```python
from build123d import *

# Parameters (mm, degrees)
CUT_EXTRUDE_1_DEPTH    = 6.35
CUT_EXTRUDE_START      = -12.7
CUT_EXTRUDE_2_DEPTH    = 12.7
HOLE_WIZARD_M2_1_D     = 2.3876
HOLE_WIZARD_M2_1_DEPTH = 4.7752
CHAMFER_1_SIZE         = 0.7874


with BuildPart() as part:
    # 스케치1 → 회전1 (revolve)
    with BuildSketch(Plane.XY, mode=Mode.PRIVATE) as revolve_1_sk:
        with BuildLine():
            Line((6.35, 38.1), (0, 38.1))
            Line((0, 38.1), (0, 0))
            Line((0, 0), (9.525, 0))
            Line((9.525, 0), (9.525, 13.263233373))
            ThreePointArc((9.525, 13.263233373), (9.110100453, 15.210106507), (7.9375, 16.818666364))
            ThreePointArc((7.9375, 16.818666364), (6.764899547, 18.42722622), (6.35, 20.374099354))
            Line((6.35, 20.374099354), (6.35, 38.1))
        make_face()
    revolve(revolve_1_sk.sketch.rotate(Axis((0, 38.1, 0), (0, -1, 0)), 270), axis=Axis((0, 38.1, 0), (0, -1, 0)))

    # 스케치2 → 컷-돌출1 (cut)
    with BuildSketch(Plane(origin=(0, 38.1, 0), x_dir=(-1, 0, 0), z_dir=(0, 1, 0))):
        with BuildLine():
            Line((-4.7498, -4.214486915), (-4.7498, 4.214486915))
            ThreePointArc((-4.7498, 4.214486915), (-6.35, 0), (-4.7498, -4.214486915))
        make_face()
    extrude(amount=-CUT_EXTRUDE_1_DEPTH, mode=Mode.SUBTRACT)

    # 스케치3 → 컷-돌출2 (cut)
    with BuildSketch(Plane.XZ.offset(CUT_EXTRUDE_START)):
        with BuildLine():
            Line((4.7498, -4.214486915), (4.7498, 4.214486915))
            ThreePointArc((4.7498, 4.214486915), (-6.35, 0), (4.7498, -4.214486915))
        make_face()
    extrude(amount=CUT_EXTRUDE_2_DEPTH, mode=Mode.SUBTRACT)

    # M2 여유 구멍1
    with Locations(Plane.ZY.offset(-4.7498)):
        with Locations((0, 6.35)):
            Hole(HOLE_WIZARD_M2_1_D / 2, depth=HOLE_WIZARD_M2_1_DEPTH)

    # 모따기1
    chamfer_1_edges = [part.edges().sort_by_distance(p)[0] for p in [
        (-5.791566796, 38.1, 2.603892095),
    ]]
    chamfer(chamfer_1_edges, length=CHAMFER_1_SIZE)


solid = part.part
```
Design review of the part built by this model. Coordinates are the model's own, in mm. A direction names the side the tool comes from. Coordinates: 2 decimals unless noted, no trailing zeros. Order: outer loops, then holes, each group sorted by start corner. A loop starts at its lowest first (then second) coordinate and runs counter-clockwise, first axis right, second up.
1) Mouldability with a two-part tool opening along Z and no side actions: class faces 5 (the flat face through (4.75, 5, 0)), 6 (the conical face through (-5.7, 37.96, 0.21)), 7 (the flat face through (-2, 0, 6.2)), 8 (the cylindrical face through (-6.346, 6.439, 0.215)) as +Z half, -Z half, draft (parallel to the pull), parting line (faces both ways), or undercut.
2) For faces 1 (the flat face through (-1, 12.7, 0)), 2 (the flat face through (4.75, 35, 0)), 3 (the cylindrical face through (-6.2, 28.96, 1.38)), 4 (the cylindrical face through (7.171, 5.185, 0.259)), list the 3-axis set-ups (+Z, -Z, +X, -X, +Y, -Y) from which the entire face can be reached by the end or side of a thin tool; tool diameter is ignored.
3) Take a section at A-A, the plane y = 25. Give the boundary of the cut face in (x, z).
4) Wall thickness on line 1 along Z through (x, y) = (-0.25, 3); line 2 along Y through (x, z) = (6, 1); line 3 along Z through (x, y) = (4.5, 2): over which ranges is each line inside the solid? List them lowest first.
5) Take a section at B-B, the plane y = 10. Give the boundary of the cut face in (x, z) (3 decimals).
6) Clearance check with flat-ended pins moving along their axes: pin 1 (1 mm diameter, centred on x = 6, y = 21, fed in from -Z); pin 2 (10 mm diameter, centred on y = 31.5, z = 0.5, fed in from -X); pin 3 (1.5 mm diameter, centred on x = -1, y = 26, fed in from -Z). State where each tip first meets the part, or that it passes through.
Returned:
1. face 5: undercut
1. face 6: parting line
1. face 7: draft
1. face 8: undercut
2. face 1: -Y
2. face 2: +Z, -Z, +X, +Y
2. face 3: +Y
2. face 4: +X
3. outline: circle Ø12.7 at (0, 0)
4. line 1: z = -9.52 to -6.35, 6.35 to 9.52
4. line 2: y = 0 to 5.7, 7 to 31.75
4. line 3: z = -8.39 to -4.48, 4.48 to 8.39
5. outline: circle Ø19.05 at (0, 0); hole (4.75, -4.214) - (4.75, 4.214) arc R6.35 ccw (long way) to start
6. pin 1: stops at z = -3.17
6. pin 2: stops at x = -6.35
6. pin 3: stops at z = -6.35
